```python
from build123d import *

# Parameters (mm, degrees)
F0_R        = 6.25
F1_DEPTH    = 25
F2_DEPTH    = 15
F0_R_2      = 3.75
F3_DEPTH    = 7.5
F4_T2_ANGLE = 359.64


# Not quite as in the source:
# - a fillet or chamfer that OpenCascade refuses, or shapes differently, is made with other operations: its cross-section is extruded or revolved along the edge and cut away or added


with BuildPart() as f1:
    # F0 (on Top) → F1 (new body)
    with BuildSketch(Plane.XY):
        with BuildLine():
            ThreePointArc((-20.8125196211, -8.5595397618), (-18.3005664883, -4.6032795782), (-17.4220903611, 0))
            ThreePointArc((-17.4220903611, 0), (-18.1998915609, 4.3405132519), (-20.4364992075, 8.1408574773))
            ThreePointArc((-20.4364992075, 8.1408574773), (-42.4189230977, 0.2813743978), (-20.8125196211, -8.5595397618))
        make_face()
        with Locations((-29.9220903611, 0)):
            Circle(F0_R, mode=Mode.SUBTRACT)
    extrude(amount=F1_DEPTH)

    # F0 (on Top) → F2 (join)
    with BuildSketch(Plane.XY):
        with BuildLine():
            ThreePointArc((-20.4364992075, 8.1408574773), (-18.1998915609, 4.3405132519), (-17.4220903611, 0))
            ThreePointArc((-17.4220903611, 0), (-18.3005664883, -4.6032795782), (-20.8125196211, -8.5595397618))
            Line((-20.8125196211, -8.5595397618), (16.7775256305, -6.2798766695))
            ThreePointArc((16.7775256305, -6.2798766695), (13.3788672096, -0.1198442426), (16.5789499879, 6.1456444673))
            Line((16.5789499879, 6.1456444673), (-20.4364992075, 8.1408574773))
        make_face()
    extrude(amount=F2_DEPTH)

    # F0 (on Top) → F3 (join)
    with BuildSketch(Plane.XY):
        with BuildLine():
            ThreePointArc((28.3779096389, 0), (24.3425743137, 6.651774101), (16.5789499879, 6.1456444673))
            ThreePointArc((16.5789499879, 6.1456444673), (13.3788672096, -0.1198442426), (16.7775256305, -6.2798766695))
            ThreePointArc((16.7775256305, -6.2798766695), (24.4484222028, -6.5955621467), (28.3779096389, 0))
        make_face()
        with Locations((20.8779096389, 0)):
            Circle(F0_R_2, mode=Mode.SUBTRACT)
    extrude(amount=F3_DEPTH)

    # F4: fillet of radius 10.139696962 on 1 edges, made by hand

    # F4_s1 → F4_t2 (revolve, cut)
    with BuildSketch(Plane(origin=(0.0034409593, -0.268007829, 0), x_dir=(0, 0, 1), z_dir=(-0.0128379671, 0.9999175899, 0))):
        with BuildLine():
            ThreePointArc((15, 38.1662582623), (12.909501189, 31.999908969), (7.5, 28.3761890884))
            Line((7.5, 28.3761890884), (15, 28.3761890884))
            Line((15, 28.3761890884), (15, 38.1662582623))
        make_face()
    revolve(axis=Axis((20.8779096389, 0, 15), (0, 0, -1)), revolution_arc=F4_T2_ANGLE, mode=Mode.SUBTRACT)


solid = f1.part
```
Could you check a few things on this model? Use its own coordinates, in mm. A direction names the side the tool comes from. Give positions to 0.01 mm unless a question says otherwise; leave off trailing zeros. Loops run counter-clockwise (first coordinate to the right, second up) from the corner with the lowest first, then second, coordinate; pieces in that order, holes last. Notation, with made-up numbers: (86.25, 54) - (116.25, 54) arc R25 cw to (116.25, 81) - close; hole circle Ø6 at (0, 6). An arc over 180 degrees is marked (long way). Use one line per item in the form item = value.
1. I want a section at A-A (x = -33.5). Please give me the cut outline in (y, z).
Response values:
outline = (-11.98, 0) - (-5.12, 0) - (-5.12, 25) - (-11.98, 25) - close; (5.12, 0) - (11.98, 0) - (11.98, 25) - (5.12, 25) - close
2. I'm going to push flat-ended pins straight in: pin 1 Ø10 at (x, z) = (-11.5, 14.5) entering from -Y; pin 2 Ø4.5 at (x, y) = (18, -2) entering from +Z; pin 3 Ø5 at (x, z) = (-15.5, 8.5) entering from +Y; pin 4 Ø1.5 at (x, z) = (5, 16.5) entering from +Y. Where does each tip first touch, or does it pass through?
Response values:
pin_1 = -8.3
pin_2 = 7.5
pin_3 = 8.01
pin_4 = through
3. I want a section at C-C (z = 18.5). Please give me the cut outline in (x, y), and give its area (3 significant figures).
Response values:
outline = circle Ø25 at (-29.92, 0); hole circle Ø12.5 at (-29.92, 0)
area = 368 mm²
4. On a 3-axis mill with a long thin cutter (end or side, diameter ignored), from which of +Z, -Z, +X, -X, +Y, -Y can I reach the whole of each face in a straight line? I mean faces 3 (the face through (-2.281, -7.436, 7.395)), 4 (the face through (-36, -3, 25)), 5 (the face through (17, -2, 7.5)). Say none if no direction works.
Response values:
face_3 = +Z, -Z, -Y
face_4 = +Z, +X, -X, +Y, -Y
face_5 = +Z, +X
5. I need wall thicknesses on probe 1 along Z at (x, y) = (3, 0.75); probe 2 along Z at (x, y) = (16.5, 5); probe 3 along Y at (x, z) = (-21.5, 9.75). Which ranges of each line are inside material? Lowest first, please.
Response values:
probe_1 = 0 to 15
probe_2 = 0 to 7.5
probe_3 = -9.24 to 9.24
6. I want a section at B-B (z = 3.5). Please give me the cut outline in (x, y), and give its area (3 significant figures).
Response values:
outline = (-20.81, -8.56) - (16.78, -6.28) arc R7.5 ccw (long way) to (16.58, 6.15) - (-20.44, 8.14) arc R12.5 ccw (long way) to start; hole circle Ø12.5 at (-29.92, 0); hole circle Ø7.5 at (20.88, 0)
area = 978 mm²
7. Thinking about a two-plate mould opening in X: for faces 1 (the face through (-1.67, 7.13, 7.4)), 2 (the face through (-8, 0, 0)), which applies, released by +X, released by -X, zero draft, split by the parting line, or undercut?
Response values:
face_1 = undercut
face_2 = zero draft
8. I want a section at D-D (x = 23). Please give me the cut outline in (y, z).
Response values:
outline = (-7.19, 0) - (-3.09, 0) - (-3.09, 7.5) - (-7.19, 7.5) - close; (3.09, 0) - (7.19, 0) - (7.19, 7.5) - (3.09, 7.5) - close
